from build123d import *

# Parameters (mm, degrees)
F0_W     = 100
F0_H     = 2200
F1_DEPTH = 100
F2_W     = 30
F2_H     = 2200
F3_DEPTH = 20
F4_W     = 40
F4_H     = 20
F5_DEPTH = 100
F6_W     = 40
F6_H     = 20
F7_DEPTH = 100


with BuildPart() as f1:
    # F0 (on Front) → F1 (new body)
    with BuildSketch(Plane.XZ):
        with Locations((50, 1100)):
            Rectangle(F0_W, F0_H)
    extrude(amount=F1_DEPTH)

    # F2 (on face) → F3 (cut)
    with BuildSketch(Plane.XZ.offset(100)):
        with Locations((15, 1100)):
            Rectangle(F2_W, F2_H)
        with Locations((85, 1100)):
            Rectangle(F2_W, F2_H)
    extrude(amount=-F3_DEPTH, mode=Mode.SUBTRACT)

    # F4 (on face) → F5 (cut)
    with BuildSketch(Plane.XY.offset(2200)):
        Polygon((20, -80), (20, -20), (80, -20), (80, -80), (100, -80), (100, 0), (0, 0), (0, -80), align=None)
        with Locations((50, -90)):
            Rectangle(F4_W, F4_H)
    extrude(amount=-F5_DEPTH, mode=Mode.SUBTRACT)

    # F6 (on face) → F7 (cut)
    with BuildSketch(Plane(origin=(0, 0, 0), x_dir=(1, 0, 0), z_dir=(0, 0, -1))):
        Polygon((80, 80), (80, 20), (20, 20), (20, 80), (0, 80), (0, 0), (100, 0), (100, 80), align=None)
        with Locations((50, 90)):
            Rectangle(F6_W, F6_H)
    extrude(amount=-F7_DEPTH, mode=Mode.SUBTRACT)


solid = f1.part
Input: part model. Units: mm. Frame: model coordinates. A direction names the side the tool comes from. Give positions to 0.01 mm unless a question says otherwise; leave off trailing zeros. Order: outer loops, then holes, each group sorted by start corner. A loop starts at its lowest first (then second) coordinate and runs counter-clockwise, first axis right, second up. Notation, with made-up numbers: M 68.25,68.25 L 83.25,68.25 A17 ccw 83.25,78.25 Z; hole C 60,-21.5 d3. An arc over 180 degrees is marked long. Answer as a JSON object with one key per item and string values.
1. Cut plane B-B, the plane y = -42. Output: boundary loops of the cut face in (x, z).
Result sheet:
{"outline": "M 0,100 L 20,100 L 20,0 L 80,0 L 80,100 L 100,100 L 100,2100 L 80,2100 L 80,2200 L 20,2200 L 20,2100 L 0,2100 Z"}
2. First-contact query: P1, Ø10, axis at y = -94.5, z = 1370.5, coming from the -X side; P2, Ø18, axis at y = -60, z = 37.5, coming from the +X side; P3, Ø16, axis at x = 57.5, y = -91, coming from the -Z side. Flat tips, straight axial feed; report the tip coordinate or a pass-through.
Result sheet:
{"P1": "x = 30", "P2": "x = 80", "P3": "z = 100"}
3. Cut plane A-A, the plane z = 1075. Output: boundary loops of the cut face in (x, y).
Result sheet:
{"outline": "M 0,-80 L 30,-80 L 30,-100 L 70,-100 L 70,-80 L 100,-80 L 100,0 L 0,0 Z"}
4. Ray query, line 1 (Y direction, x = 6, z = 1477); line 2 (Z direction, x = 90.5, y = -69.5); line 3 (X direction, y = -88, z = 1813). Return the intervals inside material, ascending. Write a range as [from, to].
Result sheet:
{"line 1": "[-80, 0]", "line 2": "[100, 2100]", "line 3": "[30, 70]"}
5. Reachability of faces 1 (the flat face through (50, -20, 2151)), 2 (the flat face through (80, -50, 49)), 3 (the flat face through (50, -20, 49)), 4 (the flat face through (80, -50, 2151)), 5 (the flat face through (20, -50, 2151)) from +Z, -Z, +X, -X, +Y, -Y: full face, straight path, thin tool, end or side. Return the list, or none.
Result sheet:
{"face 1": "+Z, +X, -X, +Y", "face 2": "-Z, +X, +Y, -Y", "face 3": "-Z, +X, -X, +Y", "face 4": "+Z, +X, +Y, -Y", "face 5": "+Z, -X, +Y, -Y"}
